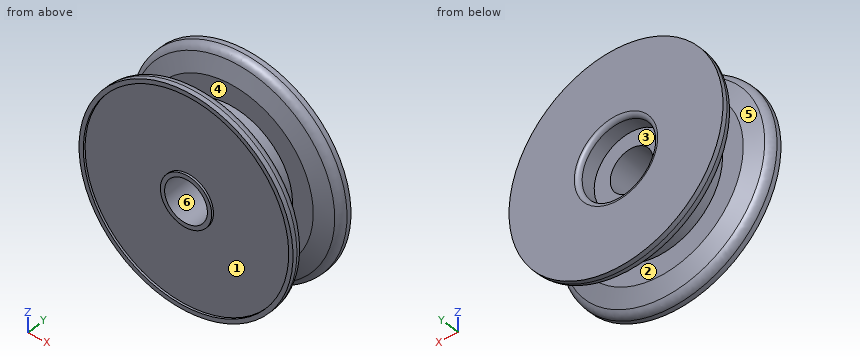
```python
from build123d import *

# Parameters (mm, degrees)
F2_R = 2.54
F3_R = 1.27


with BuildPart() as f1:
    # F0 (on Right) → F1 (revolve)
    with BuildSketch(Plane.YZ):
        Polygon((-7.916564, 6.35), (7.171036, 6.35), (7.171036, 11.1125), (12.733636, 11.1125), (12.733636, 31.75), (9.558636, 31.75), (7.171036, 25.190123), (7.171036, 19.05), (-2.353964, 19.05), (-2.353964, 25.190123), (-4.741564, 31.75), (-7.916564, 31.75), (-7.916564, 30.48), (-7.281564, 30.48), (-7.281564, 7.62), (-7.916564, 7.62), align=None)
    revolve(axis=Axis((0, 2.81315, 0), (0, 1, 0)))

    # F2
    f2_edges = [f1.edges().sort_by_distance(p)[0] for p in [
        (0, 9.558636, -31.75),
        (0, -4.741564, -31.75),
    ]]
    fillet(f2_edges, radius=F2_R)

    # F3
    f3_edges = [f1.edges().sort_by_distance(p)[0] for p in [
        (0, 12.733636, -11.1125),
    ]]
    fillet(f3_edges, radius=F3_R)


solid = f1.part
```
Source: CAD feature listing. Evaluate the final solid. Frame: model axes, mm. Face numbers are marked on the shaded views. A direction names the side the tool comes from. Give positions to 0.01 mm unless a question says otherwise; leave off trailing zeros. Loops run counter-clockwise (first coordinate to the right, second up) from the corner with the lowest first, then second, coordinate; pieces in that order, holes last. Notation, with made-up numbers: (-14, 9) - (-8, 9) arc R20 ccw to (-8, 17) - close; hole circle Ø5 at (72, 39.25). An arc over 180 degrees is marked (long way). Use CSV: the item, a comma, the result in double quotes.
1) Pin query (flat end, axial travel): P1, Ø6, axis at x = -9.5, y = -2, coming from the -Z side; P2, Ø11, axis at x = 3, z = -0.5, coming from the +Y side; P3, Ø5, axis at y = 9.5, z = -9, coming from the -X side. Return the tip coordinate at first contact, or that it passes through.
Worked out:
P1,"stops at z = -29.92"
P2,"stops at y = 7.17"
P3,"stops at x = -30.95"
2) Mould query, pull axis Z, two halves, no side actions, for the marked faces 4, 5 and 6. Classes: +Z half, -Z half, draft (parallel to the pull), parting line (faces both ways), or undercut.
Worked out:
face 4,"draft"
face 5,"parting line"
face 6,"undercut"
3) Set-up query: the marked faces 1, 2 and 3. Return all of +Z, -Z, +X, -X, +Y, -Y with unobstructed straight access to the full face (end or side cutting, diameter ignored); none if empty.
Worked out:
face 1,"-Y"
face 2,"none"
face 3,"+Y"
4) Line query: line 1 (X direction, y = -7.45, z = 0); line 2 (Y direction, x = -15.5, z = -16); line 3 (X direction, y = 2, z = 0). Output: solid intervals per line, ascending.
Worked out:
line 1,"x = -31.75 to -30.48, -7.62 to -6.35, 6.35 to 7.62, 30.48 to 31.75"
line 2,"y = -7.28 to -2.35, 7.17 to 12.73"
line 3,"x = -19.05 to -6.35, 6.35 to 19.05"
5) Cut plane A-A (y = -3.25). Output: boundary loops of the cut face in (x, z), and give its area (3 significant figures).
Worked out:
outline,"circle Ø55.3 at (0, 0); hole circle Ø12.7 at (0, 0)"
area,"2,280 mm^2"
